Verification items for the finished model (mm, model axes). Coordinates: 2 decimals unless noted, no trailing zeros. Loops run counter-clockwise (first coordinate to the right, second up) from the corner with the lowest first, then second, coordinate; pieces in that order, holes last. Notation, with made-up numbers: (-31, -24) -> (-21, -24) arc R28 ccw to (-21, -1) -> close; hole circle Ø2 at (-34.75, 36). An arc over 180 degrees is marked (long way). Answer as a JSON object with one key per item and string values. Group by question number.
Q1. Scan lines: L1, parallel to Y at x = 0, z = 1.1; L2, parallel to X at y = 31, z = 1.15; L3, parallel to Y at x = 0.25, z = 0.6. Record each from-to range of solid material in increasing order.
Q2. Cross-section at B-B on z = 1.05. Give the number of separate pieces and of enclosed holes in the cut face, and give its area (3 significant figures).
Q3. Cross-section at C-C on y = 13. Record the boundary of the cut face in (x, z), and give its area (3 significant figures).
Q4. Cross-section at A-A on x = -3.25. Record the boundary of the cut face in (y, z), and give its area (3 significant figures).
Q5. Cross-section at D-D on x = -6.5. Record the boundary of the cut face in (y, z), and give its area (3 significant figures).
Q6. Gauge pin test, flat end, axial feed: pin 1 Ø2.5 at (x, y) = (0.2, 24.05) entering from -Z. Record the tip position at first contact, or that the pin passes through.
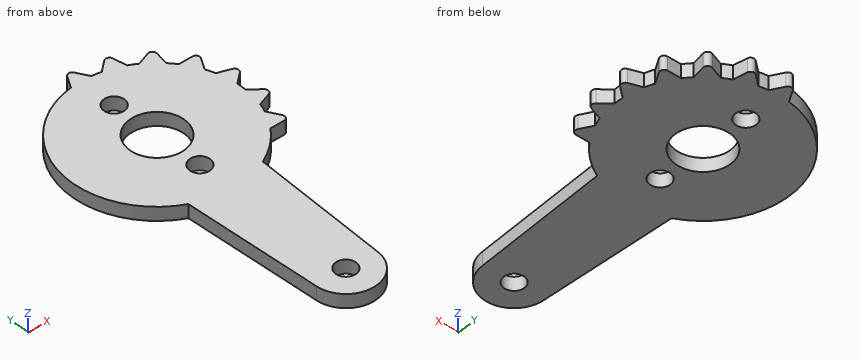
```python
from build123d import *

# Parameters (mm, degrees)
SKETCH1_R           = 4
SKETCH1_R_2         = 1.5
BOSS_EXTRUDE1_DEPTH = 2


with BuildPart() as part:
    # Sketch1 → Boss-Extrude1 (new body)
    with BuildSketch(Plane.XY):
        with BuildLine():
            Line((-5.322767432, 19.832757644), (-4.500006862, -0.184957582))
            ThreePointArc((-4.500006862, -0.184957582), (-0.000167017, -4.503806283), (4.499993132, -0.185291335))
            Line((4.499993132, -0.185291335), (5.67721776, 19.814708665))
            ThreePointArc((5.67721776, 19.814708665), (8.148561948, 21.404983206), (10.180318916, 23.528301089))
            Line((10.180318916, 23.528301089), (12.180312779, 23.523346368))
            ThreePointArc((12.180312779, 23.523346368), (12.679597114, 23.812434692), (12.680312779, 24.389371772))
            Line((12.680312779, 24.389371772), (11.684612917, 26.123898158))
            ThreePointArc((11.684612917, 26.123898158), (11.934719035, 26.754030681), (12.150293859, 27.396796239))
            Line((12.150293859, 27.396796239), (14.031367948, 28.076178512))
            ThreePointArc((14.031367948, 28.076178512), (14.401667723, 28.518597977), (14.205016126, 29.060986265))
            Line((14.205016126, 29.060986265), (12.67612135, 30.350358501))
            ThreePointArc((12.67612135, 30.350358501), (12.695626208, 31.028030714), (12.678361511, 31.705763698))
            Line((12.678361511, 31.705763698), (14.213630529, 32.987539436))
            ThreePointArc((14.213630529, 32.987539436), (14.410282126, 33.529927724), (14.039982351, 33.972347189))
            Line((14.039982351, 33.972347189), (12.162299935, 34.661047954))
            ThreePointArc((12.162299935, 34.661047954), (11.948850959, 35.304522586), (11.700829119, 35.935478396))
            Line((11.700829119, 35.935478396), (12.705116964, 37.665046528))
            ThreePointArc((12.705116964, 37.665046528), (12.704401299, 38.241983607), (12.205116964, 38.531071932))
            Line((12.205116964, 38.531071932), (10.205123119, 38.536033749))
            ThreePointArc((10.205123119, 38.536033749), (9.784465406, 39.067698263), (9.335601516, 39.575774317))
            Line((9.335601516, 39.575774317), (9.687776253, 41.5445234))
            ThreePointArc((9.687776253, 41.5445234), (9.489779645, 42.086422145), (8.92173181, 42.18731101))
            Line((8.92173181, 42.18731101), (7.040655311, 41.507935412))
            ThreePointArc((7.040655311, 41.507935412), (6.463526388, 41.863663221), (5.867960059, 42.187578047))
            Line((5.867960059, 42.187578047), (5.525544216, 44.158047887))
            ThreePointArc((5.525544216, 44.158047887), (5.154147979, 44.59954731), (4.585851596, 44.500068031))
            Line((4.585851596, 44.500068031), (3.050578029, 43.21829774))
            ThreePointArc((3.050578029, 43.21829774), (2.386588163, 43.355182821), (1.716153483, 43.455867511))
            Line((1.716153483, 43.455867511), (0.720447466, 45.190390364))
            ThreePointArc((0.720447466, 45.190390364), (0.220447466, 45.47823912), (-0.279552534, 45.190390364))
            Line((-0.279552534, 45.190390364), (-1.283846517, 43.460825796))
            ThreePointArc((-1.283846517, 43.460825796), (-12.125641313, 33.154858755), (-5.322767432, 19.832757644))
        make_face()
        with Locations((0.19564328, 31.048690205)):
            Circle(SKETCH1_R, mode=Mode.SUBTRACT)
        with Locations((0.19564328, 38.048690205)):
            Circle(SKETCH1_R_2, mode=Mode.SUBTRACT)
        with Locations((0.19564328, 24.048690205)):
            Circle(SKETCH1_R_2, mode=Mode.SUBTRACT)
        Circle(SKETCH1_R_2, mode=Mode.SUBTRACT)
    extrude(amount=BOSS_EXTRUDE1_DEPTH)


solid = part.part
```
Computed values:
{
 "1": {"L1": "y = -4.5 to -1.5, 1.5 to 22.56, 25.54 to 27.05, 35.04 to 36.56, 39.54 to 45.43", "L2": "x = -12.3 to -3.8, 4.2 to 12.7", "L3": "y = -4.5 to -1.48, 1.48 to 22.55, 25.55 to 27.05, 35.05 to 36.55, 39.55 to 45.48"},
 "2": {"separate pieces": "1", "enclosed holes": "4", "area": "665 mm²"},
 "3": {"outline": "(-5.04, 0) -> (5.28, 0) -> (5.28, 2) -> (-5.04, 2) -> close", "area": "20.6 mm²"},
 "4": {"outline": "(-3.12, 0) -> (29.02, 0) -> (29.02, 2) -> (-3.12, 2) -> close; (33.08, 0) -> (43.06, 0) -> (43.06, 2) -> (33.08, 2) -> close", "area": "84.2 mm²"},
 "5": {"outline": "(20.49, 0) -> (41.6, 0) -> (41.6, 2) -> (20.49, 2) -> close", "area": "42.2 mm²"},
 "6": {"pin 1": "passes through"}
}
